```python
from build123d import *

# Parameters (mm, degrees)
PAD006_DEPTH = 3
SKETCH005_R  = 8
PAD005_DEPTH = 2.3
SKETCH004_R  = 6
PAD004_DEPTH = 4
SKETCH007_R  = 1.6
PAD007_DEPTH = 15
SKETCH003_R  = 1.4
PAD003_DEPTH = 4
SKETCH002_W  = 42
SKETCH002_H  = 4
PAD002_DEPTH = 9
SKETCH001_R  = 2
PAD001_DEPTH = 42
PAD_DEPTH    = 8


with BuildPart() as nutmount:
    # Sketch006 → Pad006 (new body)
    with BuildSketch(Plane.XZ.offset(-4)):
        Polygon((5.531089, 0.5), (8.562178, 2.25), (8.562178, 5.75), (8.562178, 8), (2.5, 8), (2.5, 5.75), (2.5, 2.25), align=None)
        Polygon((39.562178, 2.25), (39.562178, 5.75), (39.562178, 8), (33.5, 8), (33.5, 5.75), (33.5, 2.25), (36.531089, 0.5), align=None)
    extrude(amount=-PAD006_DEPTH)


with BuildPart() as hotendmount:
    # Sketch005 → Pad005 (new body)
    with BuildSketch(Plane.XY):
        with Locations((14.75, 0)):
            Circle(SKETCH005_R)
    extrude(amount=PAD005_DEPTH)


with BuildPart() as springmount:
    # Sketch004 → Pad004 (new body)
    with BuildSketch(Plane.XY):
        with Locations((10.5, 42)):
            Circle(SKETCH004_R)
    extrude(amount=PAD004_DEPTH)


with BuildPart() as hotendmount02:
    # Sketch007 → Pad007 (new body)
    with BuildSketch(Plane.XZ):
        with Locations((5.5, 4)):
            Circle(SKETCH007_R)
        with Locations((36.5, 4)):
            Circle(SKETCH007_R)
    extrude(amount=-PAD007_DEPTH)


with BuildPart() as cutblock:
    # Sketch003 → Pad003 (new body)
    with BuildSketch(Plane.XZ.offset(-11)):
        with Locations((37, 13.5)):
            Circle(SKETCH003_R)
        with BuildLine():
            ThreePointArc((5, 14.9), (3.6, 13.5), (5, 12.1))
            Line((5, 12.1), (7, 12.1))
            ThreePointArc((7, 12.1), (8.4, 13.5), (7, 14.9))
            Line((5, 14.9), (7, 14.9))
        make_face()
    extrude(amount=-PAD003_DEPTH)

    # Fusion001: union NutMount, HotEndMount, SpringMount, HotEndMount02
    add(nutmount.part)
    add(hotendmount.part)
    add(springmount.part)
    add(hotendmount02.part)


with BuildPart() as pad002:
    # Sketch002 → Pad002 (new body)
    with BuildSketch(Plane.XY.offset(8)):
        with Locations((21, 13)):
            Rectangle(SKETCH002_W, SKETCH002_H)
    extrude(amount=PAD002_DEPTH)


with BuildPart() as pad001:
    # Sketch001 → Pad001 (new body)
    with BuildSketch(Plane.YZ):
        with Locations((26, 4)):
            Circle(SKETCH001_R)
    extrude(amount=PAD001_DEPTH)


with BuildPart() as final:
    # Sketch → Pad (new body)
    with BuildSketch(Plane.XY):
        with BuildLine():
            Line((0, 50), (42, 50))
            Line((42, 50), (42, 0))
            Line((20.35, 0), (42, 0))
            ThreePointArc((20.35, 0), (14.75, 5.6), (9.15, 0))
            Line((9.15, 0), (0, 0))
            Line((0, 0), (0, 50))
        make_face()
    extrude(amount=PAD_DEPTH)

    # Cut: cut Pad001
    add(pad001.part, mode=Mode.SUBTRACT)

    # Fusion: union Pad002
    add(pad002.part)

    # Cut001: cut CutBlock
    add(cutblock.part, mode=Mode.SUBTRACT)


solid = final.part
```
For this review, take the finished solid that the model builds, in its own axes (mm). A direction names the side the tool comes from. Round coordinates to 2 decimals unless told otherwise and drop trailing zeros. Write each loop counter-clockwise with the first axis right and the second up, starting at its lowest first coordinate (ties: lowest second). Pieces come first, ordered by that corner, then holes.
1) Take a section at B-B on x = 31. Give the boundary of the cut face in (y, z), then the cut area to 3 significant figures.
Answer below:
outline: (0, 0) - (50, 0) - (50, 8) - (15, 8) - (15, 17) - (11, 17) - (11, 8) - (0, 8) - close; hole circle Ø4 at (26, 4)
area: 423 mm2
2) Take a section at D-D on y = 42. Give the boundary of the cut face in (x, z).
Answer below:
outline: (0, 0) - (4.5, 0) - (4.5, 4) - (16.5, 4) - (16.5, 0) - (42, 0) - (42, 8) - (0, 8) - close
3) Machinability: for faces 4 (the face through (14.9, 8, 1.1)), 5 (the face through (21, 6, 8)), 6 (the face through (8.562, 5, 5)), which of the approach directions +Z, -Z, +X, -X, +Y, -Y give a long, thin tool a straight path to every point of the face, cutting with its end or side? Answer none if there is none.
Answer below:
face 4: -Z, -Y
face 5: +Z, +X, -X, -Y
face 6: +Z
4) For line 1 along Z through (x, y) = (36.5, 11.75); line 2 along X through (y, z) = (11, 2.75); line 3 along Y through (x, z) = (21, 10), list the stretches that pass through material, from the lowest coordinate up.
Answer below:
line 1: z = 0 to 2.4, 5.6 to 12.19, 14.81 to 17
line 2: x = 0 to 4.5, 6.5 to 35.5, 37.5 to 42
line 3: y = 11 to 15
5) Take a section at A-A on z = 13.5. Give the boundary of the cut face in (x, y).
Answer below:
outline: (0, 11) - (3.6, 11) - (3.6, 15) - (0, 15) - close; (8.4, 11) - (35.6, 11) - (35.6, 15) - (8.4, 15) - close; (38.4, 11) - (42, 11) - (42, 15) - (38.4, 15) - close
6) Take a section at C-C on y = 26. Give the boundary of the cut face in (x, z), then the cut area to 3 significant figures.
Answer below:
outline: (0, 0) - (42, 0) - (42, 2) - (0, 2) - close; (0, 6) - (42, 6) - (42, 8) - (0, 8) - close
area: 168 mm2
7) Mouldability with a two-part tool opening along Z and no side actions: class faces 1 (the face through (21, 13, 17)), 2 (the face through (33.5, 5, 5)), 3 (the face through (8.4, 13, 13.5)) as +Z half, -Z half, draft (parallel to the pull), parting line (faces both ways), or undercut.
Answer below:
face 1: +Z half
face 2: draft
face 3: undercut
8) Insertion check: pin 1 Ø1.8 at (x, z) = (38, 3.5) entering from -Y; pin 2 Ø1.5 at (x, y) = (24, 40.5) entering from +Z; pin 3 Ø5 at (y, z) = (40.5, 12) entering from -X; pin 4 Ø3 at (x, z) = (36.5, 4) entering from -Y. Each pin has a flat end and moves straight along its axis. Give the tip position at first contact, or say it passes through.
Answer below:
pin 1: stops at y = 0
pin 2: stops at z = 8
pin 3: passes through
pin 4: stops at y = 15
